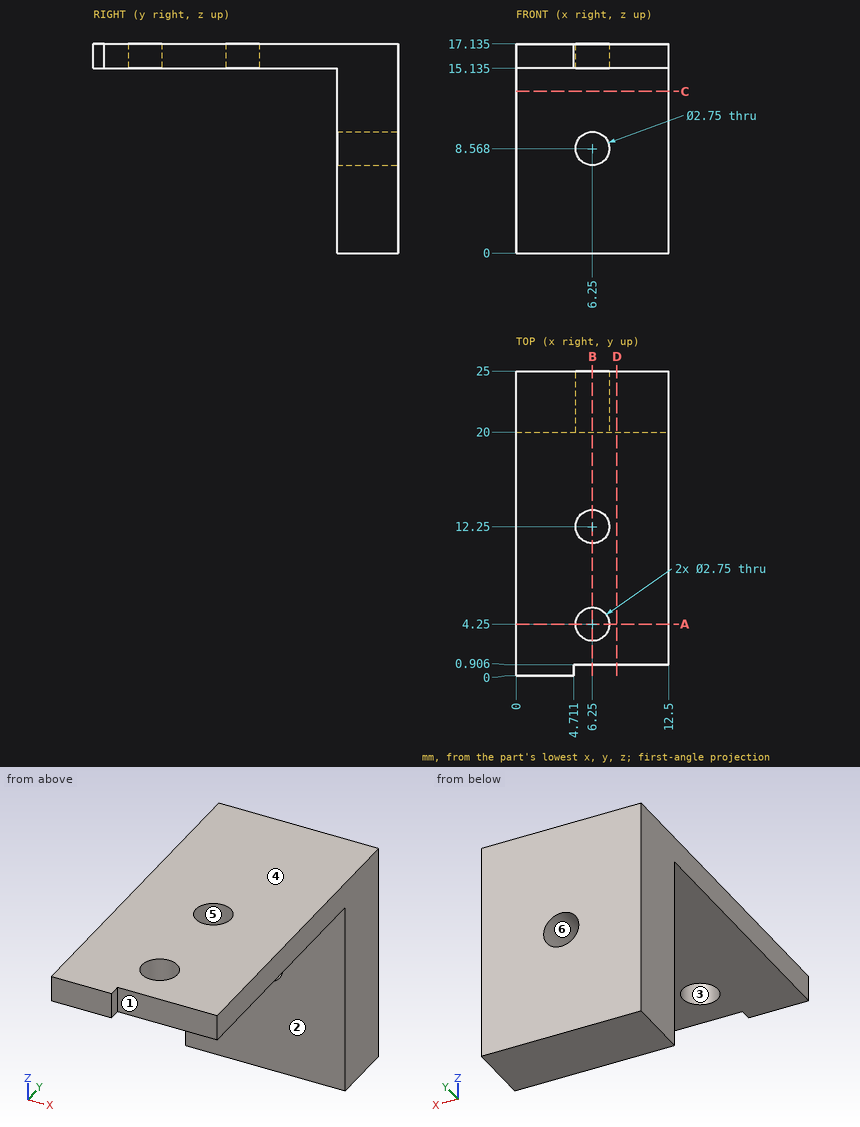
Design review of the part shown in the three views and the two pictorial views. Dimensions are in mm from the part's minimum x, y and z. A direction names the side the tool comes from. Give positions to 0.01 mm unless a question says otherwise; leave off trailing zeros. Write each loop counter-clockwise with the first axis right and the second up, starting at its lowest first coordinate (ties: lowest second). Pieces come first, ordered by that corner, then holes. Notation, with made-up numbers: M 84.5,84 L 140.5,84 A16 cw 140.5,113 Z; hole C 25,74.25 d11. An arc over 180 degrees is marked long. Return JSON: item names as keys, results as strings. Group by question number.
Item 1: Take a section at D-D (x = 8.25). Give the boundary of the cut face in (y, z) (1 decimal).
Item 2: Take a section at C-C (z = 13.25). Give the boundary of the cut face in (x, y).
Item 3: The part is to be moulded in two halves that separate along Z. For the marked faces 4, 5 and 6, say which applies: pulls with the +Z half, pulls with the -Z half, needs draft (parallel to the pull), parting line crosses it, or undercut.
Item 4: Tool access review of the marked faces 1, 2 and 3: name each direction out of +Z, -Z, +X, -X, +Y, -Y from which nothing blocks a thin tool from reaching the whole face with its end or side.
Item 5: Wall thickness on line 1 along Y through (x, z) = (6.25, 16.25) (1 decimal); line 2 along Z through (x, y) = (6.25, 21.4) (1 decimal); line 3 along Z through (x, y) = (4, 2.5) (1 decimal): over which ranges is each line inside the solid? List them lowest first.
Item 6: Take a section at B-B (x = 6.25). Give the boundary of the cut face in (y, z) (1 decimal).
Item 7: Take a section at A-A (y = 4.25). Give the boundary of the cut face in (x, z) (1 decimal), plus the area to 3 significant figures.
Item 8: Clearance check with flat-ended pins moving along their axes: pin 1 Ø1.6 at (x, z) = (6.25, 8.57) entering from +Y; pin 2 Ø6 at (x, y) = (5.5, 7) entering from -Z (1 decimal); pin 3 Ø0.6 at (x, z) = (8.5, 15.5) entering from -Y. State where each tip first meets the part, or that it passes through.
Return value:
{
 "1": {"outline": "M 0.9,15.1 L 20,15.1 L 20,0 L 25,0 L 25,17.1 L 0.9,17.1 Z"},
 "2": {"outline": "M 0,20 L 12.5,20 L 12.5,25 L 0,25 Z"},
 "3": {"face 4": "pulls with the +Z half", "face 5": "needs draft", "face 6": "undercut"},
 "4": {"face 1": "+Z, -Z, +X, -Y", "face 2": "-Z, +X, -X, -Y", "face 3": "+Z, -Z"},
 "5": {"line 1": "y = 0.9 to 2.9, 5.6 to 10.9, 13.6 to 25", "line 2": "z = 0 to 7.2, 9.9 to 17.1", "line 3": "z = 15.1 to 17.1"},
 "6": {"outline": "M 0.9,15.1 L 2.9,15.1 L 2.9,17.1 L 0.9,17.1 Z; M 5.6,15.1 L 10.9,15.1 L 10.9,17.1 L 5.6,17.1 Z; M 13.6,15.1 L 20,15.1 L 20,9.9 L 25,9.9 L 25,17.1 L 13.6,17.1 Z; M 20,0 L 25,0 L 25,7.2 L 20,7.2 Z"},
 "7": {"outline": "M 0,15.1 L 4.9,15.1 L 4.9,17.1 L 0,17.1 Z; M 7.6,15.1 L 12.5,15.1 L 12.5,17.1 L 7.6,17.1 Z", "area": "19.5 mm2"},
 "8": {"pin 1": "passes through", "pin 2": "stops at z = 15.1", "pin 3": "stops at y = 0.91"}
}
